from build123d import *

# Parameters (mm, degrees)
F1_DEPTH = 25.4
F2_DEPTH = 84.1375
F3_R     = 1.5875
F4_DEPTH = 25.4
F5_R     = 2.12725
F5_R_2   = 1.5875
F6_DEPTH = 0.9525


with BuildPart() as f1:
    # F0 (on Right) → F1 (new body)
    with BuildSketch(Plane.YZ):
        Polygon((0, 4.2545), (0, 0), (19.05, 0), (19.05, 4.2545), (19.05, 17.0903187245), (19.05, 17.399), (4.699, 17.399), (4.699, 13.1445), (11.8745, 13.1445), (12.7, 11.5581387654), (12.7, 6.1031985097), (11.7745716125, 4.2545), align=None)
    extrude(amount=F1_DEPTH)

    # F2 (add): a face of the model
    f2_faces = [f1.faces().sort_by_distance(p)[0] for p in [
        (12.7, 0, 2.12725),
    ]]
    extrude(f2_faces, amount=F2_DEPTH)

    # F3 (on face) → F4 (cut)
    with BuildSketch(Plane(origin=(0, 0, 0), x_dir=(1, 0, 0), z_dir=(0, 0, -1))):
        with Locations((12.7, 58.7375)):
            Circle(F3_R)
        with Locations((12.7, 46.0375)):
            Circle(F3_R)
    extrude(amount=-F4_DEPTH, mode=Mode.SUBTRACT)

    # F5 (on face) → F6 (cut)
    with BuildSketch(Plane.XY.offset(4.2545)):
        with Locations((12.7, -46.0375)):
            Circle(F5_R)
        with Locations((12.7, -46.0375)):
            Circle(F5_R_2, mode=Mode.SUBTRACT)
        with Locations((12.7, -58.7375)):
            Circle(F5_R)
        with Locations((12.7, -58.7375)):
            Circle(F5_R_2, mode=Mode.SUBTRACT)
    extrude(amount=-F6_DEPTH, mode=Mode.SUBTRACT)


solid = f1.part
Model file for the job. Use its own axes, mm. A direction names the side the tool comes from. Coordinates: 2 decimals unless noted, no trailing zeros. Order: outer loops, then holes, each group sorted by start corner. A loop starts at its lowest first (then second) coordinate and runs counter-clockwise, first axis right, second up. Notation, with made-up numbers: (15, 84.5) -> (33, 84.5) arc R18 cw to (33, 104.5) -> close; hole circle Ø5 at (69, 0). An arc over 180 degrees is marked (long way). Return JSON: item names as keys, results as strings. Group by question number.
Item 1: Tool access for faces 5 (the flat face through (13, 8, 13.144)), 6 (the flat face through (13, 4.699, 15)), 7 (the cylindrical face through (13.682, -47.925, 3.785)), 8 (the flat face through (25.4, -21, 4)): list every direction of +Z, -Z, +X, -X, +Y, -Y with a clear straight run to the whole face (end or side of a thin tool).
Item 2: Saw through at A-A on x = 12.7. State how many separate pieces and enclosed holes the cut face has, then the cut area to 3 significant figures.
Item 3: Saw through at B-B on x = 18.5. Write the cut outline in (y, z).
Item 4: Wall check: line 1 along Y through (x, z) = (12.7, 3.8); line 2 along Z through (x, y) = (16, -27); line 3 along Z through (x, y) = (12.5, 7.5). Give the ranges that are in metal, low to high. Write a range as [from, to].
Item 5: Flat gauge pins, fed straight in: P1, Ø12.5, axis at x = 19, y = -30, coming from the +Z side; P2, Ø2.5, axis at x = 12.7, y = -58.74, coming from the -Z side; P3, Ø6, axis at y = -42.5, z = 5, coming from the -X side; P4, Ø4, axis at x = 12.7, y = -58.74, coming from the +Z side. Where does each tip first touch, or does it go through?
Item 6: Pull direction Y, two halves, no side cores. Call faces 1 (the flat face through (13, 12.7, 9)), 2 (the cylindrical face through (12.356, -57.188, 1.628)), 3 (the flat face through (13, 19.05, 9)), 4 (the flat face through (13, 12, 17.399)): pulls with the +Y half, pulls with the -Y half, needs draft (parallel to the pull), parting line crosses it, or undercut.
Item 7: Saw through at C-C on y = -15.5. Write the cut outline in (x, z), then the cut area to 3 significant figures.
Values found:
{
 "1": {"face 5": "+X, -X, -Y", "face 6": "+Z, +X, -X, -Y", "face 7": "+Z", "face 8": "+Z, -Z, +X, +Y, -Y"},
 "2": {"separate pieces": "3", "enclosed holes": "0", "area": "529 mm2"},
 "3": {"outline": "(-84.14, 0) -> (19.05, 0) -> (19.05, 17.4) -> (4.7, 17.4) -> (4.7, 13.14) -> (11.87, 13.14) -> (12.7, 11.56) -> (12.7, 6.1) -> (11.77, 4.25) -> (-84.14, 4.25) -> close"},
 "4": {"line 1": "y = [-84.14, -60.86], [-56.61, -48.16], [-43.91, 19.05]", "line 2": "z = [0, 4.25]", "line 3": "z = [0, 4.25], [13.14, 17.4]"},
 "5": {"P1": "stops at z = 4.25", "P2": "passes through", "P3": "stops at x = 0", "P4": "stops at z = 3.3"},
 "6": {"face 1": "pulls with the -Y half", "face 2": "undercut", "face 3": "pulls with the +Y half", "face 4": "needs draft"},
 "7": {"outline": "(0, 0) -> (25.4, 0) -> (25.4, 4.25) -> (0, 4.25) -> close", "area": "108 mm2"}
}
